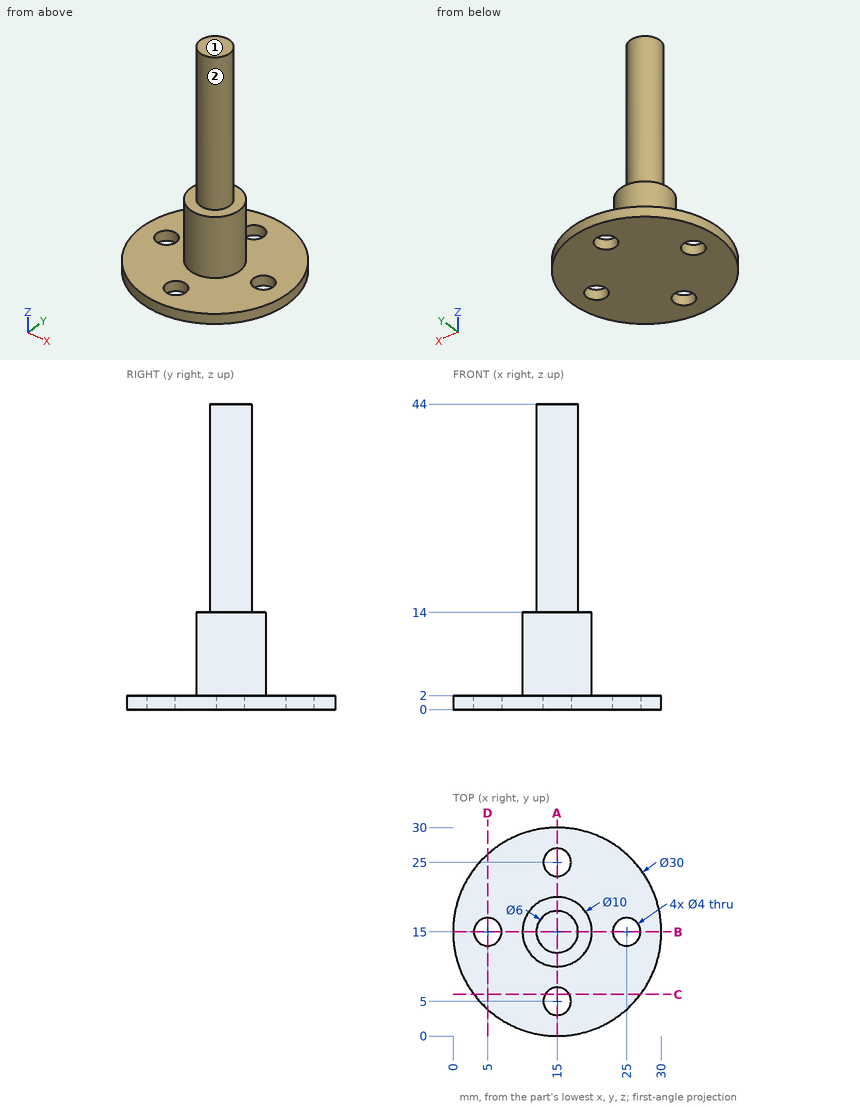
Answer from the drawing. Dimensions are ordinates in mm from the lowest x, y and z of the part. A direction names the side the tool comes from. Round coordinates to 2 decimals unless told otherwise and drop trailing zeros. Write each loop counter-clockwise with the first axis right and the second up, starting at its lowest first coordinate (ties: lowest second). Pieces come first, ordered by that corner, then holes. Notation, with made-up numbers: (55.25, -24) -> (65.25, -24) arc R22 ccw to (65.25, -3) -> close; hole circle Ø6 at (-4.75, 85.5). An arc over 180 degrees is marked (long way). Answer in a Markdown table with one row per item. Add a question column.
1) Find section A-A, the plane x = 15. Determine the outline of the cut face in (y, z).
2) Find section C-C, the plane y = 6. Determine the outline of the cut face in (x, z), and give its area (3 significant figures).
3) Given P1, Ø8, axis at x = 14, z = 12.5, coming from the +Y side; P2, Ø4, axis at x = 9.5, y = 25, coming from the +Z side; P3, Ø1.5, axis at x = 20.5, y = 14.5, coming from the +Z side, each flat-ended and moving along its own axis, determine where each tip first touches the part or whether it passes through.
4) Find section D-D, the plane x = 5. Determine the outline of the cut face in (y, z), and give its area (3 significant figures).
5) Which of the six approach directions +Z, -Z, +X, -X, +Y, -Y give full straight-line access (tool end or side, diameter ignored) to the marked faces 1 and 2?
6) Consider line 1 (Y direction, x = 15, z = 0.8); line 2 (Z direction, x = 12, y = 19.5); line 3 (Y direction, x = 5, z = 0.6). Determine where each line is inside the solid, lowest interval first.
Findings below:
| question | item | result |
|---|---|---|
| 1 | outline | (0, 0) -> (3, 0) -> (3, 2) -> (0, 2) -> close; (7, 0) -> (23, 0) -> (23, 2) -> (20, 2) -> (20, 14) -> (18, 14) -> (18, 44) -> (12, 44) -> (12, 14) -> (10, 14) -> (10, 2) -> (7, 2) -> close; (27, 0) -> (30, 0) -> (30, 2) -> (27, 2) -> close |
| 2 | outline | (3, 0) -> (13.27, 0) -> (13.27, 2) -> (3, 2) -> close; (16.73, 0) -> (27, 0) -> (27, 2) -> (16.73, 2) -> close |
| 2 | area | 41.1 mm² |
| 3 | P1 | y = 20 |
| 3 | P2 | z = 2 |
| 3 | P3 | z = 14 |
| 4 | outline | (3.82, 0) -> (13, 0) -> (13, 2) -> (3.82, 2) -> close; (17, 0) -> (26.18, 0) -> (26.18, 2) -> (17, 2) -> close |
| 4 | area | 36.7 mm² |
| 5 | face 1 | +Z, +X, -X, +Y, -Y |
| 5 | face 2 | +Z |
| 6 | line 1 | 0 to 3, 7 to 23, 27 to 30 |
| 6 | line 2 | 0 to 2 |
| 6 | line 3 | 3.82 to 13, 17 to 26.18 |
